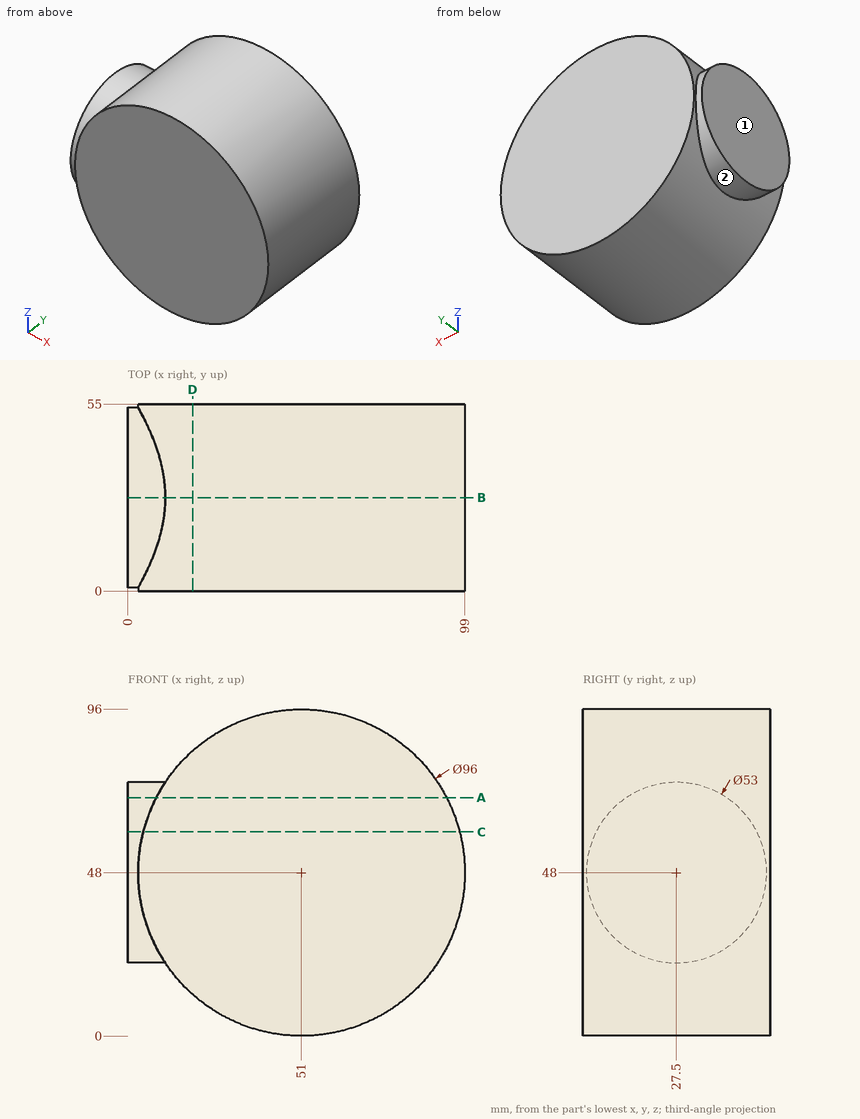
Geometry check sheet. Reference: drawing and pictorial views, mm from the part's lowest x, y, z. A direction names the side the tool comes from. Give positions to 0.01 mm unless a question says otherwise; leave off trailing zeros. Loops run counter-clockwise (first coordinate to the right, second up) from the corner with the lowest first, then second, coordinate; pieces in that order, holes last.
1. Set-up check for the marked faces 1 and 2: record each of +Z, -Z, +X, -X, +Y, -Y from which the full face is reachable in a straight line by a thin tool's end or side.
2. Thickness scan on line 1 (Z direction, x = 11, y = 14.5); line 2 (Z direction, x = 50, y = 15.5); line 3 (X direction, y = 25.5, z = 75). Record the ranges inside material, lowest first.
3. Section check B-B, the plane y = 27.5. Enter the section's corners in (x, z).
4. Go/stop test with flat-tipped pins: pin 1 Ø10 at (y, z) = (30.5, 86) entering from +X; pin 2 Ø5 at (x, y) = (53.5, 7.5) entering from -Z; pin 3 Ø2 at (x, y) = (24, 46) entering from +Z. Record where each tip stops, or that it passes through.
5. Section check D-D, the plane x = 19. Enter the section's corners in (y, z), then the cut area to 3 significant figures.
6. Section check C-C, the plane z = 60. Enter the section's corners in (x, y).
7. Section check A-A, the plane z = 70. Enter the section's corners in (x, y), then the cut area to 3 significant figures.
Geometry says:
1. face 1: +Z, -Z, -X, +Y, -Y
1. face 2: -X
2. line 1: z = 21.47 to 74.53
2. line 2: z = 0.01 to 95.99
2. line 3: x = 11.31 to 90.69
3. outline: (0, 21.5) - (10.98, 21.5) arc R48 ccw (long way) to (10.98, 74.5) - (0, 74.5) - close
4. pin 1: stops at x = 85.86
4. pin 2: stops at z = 0
4. pin 3: stops at z = 88.35
5. outline: (0, 12.22) - (55, 12.22) - (55, 83.78) - (0, 83.78) - close
5. area: 3,940 mm2
6. outline: (0, 3.87) - (4.52, 3.87) - (4.52, 0) - (97.48, 0) - (97.48, 55) - (4.52, 55) - (4.52, 51.13) - (0, 51.13) - close
7. outline: (0, 12.73) - (8.34, 12.73) - (8.34, 0) - (93.66, 0) - (93.66, 55) - (8.34, 55) - (8.34, 42.27) - (0, 42.27) - close
7. area: 4,940 mm2
